Design review of the part built by this model. Coordinates are the model's own, in mm. Coordinates: 2 decimals unless noted, no trailing zeros. Loops run counter-clockwise (first coordinate to the right, second up) from the corner with the lowest first, then second, coordinate; pieces in that order, holes last. Notation, with made-up numbers: M 84,65 L 143,65 A19 cw 143,82 Z; hole C -4.5,-18 d7. An arc over 180 degrees is marked long. One line per item, written item: value.
```python
from build123d import *

# Parameters (mm, degrees)
EXTRUDE_1_DEPTH     = 2
SKETCH_3_W          = 2
SKETCH_3_H          = 5
CUT_EXTRUDE_2_DEPTH = 10
CHAMFER_1_SIZE      = 3
SKETCH_4_W          = 16
SKETCH_4_H          = 3
CUT_EXTRUDE_3_DEPTH = 2
FILLET_1_R          = 1
FILLET_START        = -1
FILLET_2_DEPTH      = 4
FILLET_2_2_DEPTH    = 2
FILLET_3_R          = 0.5
CUT_EXTRUDE_4_DEPTH = 10
SKETCH_7_R          = 1
CUT_EXTRUDE_6_DEPTH = 10
FILLET_5_R          = 1


with BuildPart() as part:
    # 草图1 → 凸台-拉伸1 (new body)
    with BuildSketch(Plane(origin=(0, 0, 0), x_dir=(1, 0, 0), z_dir=(0, 1, 0))):
        Polygon((40, -10), (40, 0), (0, 0), (0, 5), (47.2, 5), (47.2, 0), (47.2, -10), align=None)
    extrude_1 = extrude(amount=EXTRUDE_1_DEPTH)

    # 草图3 → 切除-拉伸2 (cut)
    with BuildSketch(Plane.XZ):
        with Locations((41, 7.5)):
            Rectangle(SKETCH_3_W, SKETCH_3_H)
    cut_extrude_2 = extrude(amount=-CUT_EXTRUDE_2_DEPTH, mode=Mode.SUBTRACT)

    # 镜向1: 凸台-拉伸1, 切除-拉伸2 across plane
    add(extrude_1.mirror(Plane(origin=(0, 0, 0), x_dir=(0, 0, 1), z_dir=(1, 0, 0))))
    add(cut_extrude_2.mirror(Plane(origin=(0, 0, 0), x_dir=(0, 0, 1), z_dir=(1, 0, 0))), mode=Mode.SUBTRACT)

    # 倒角1
    chamfer_1_edges = [part.edges().sort_by_distance(p)[0] for p in [
        (47.2, 1, -5),
        (-47.2, 1, -5),
    ]]
    chamfer(chamfer_1_edges, length=CHAMFER_1_SIZE)

    # 草图4 → 切除-拉伸3 (cut)
    with BuildSketch(Plane.XZ):
        Rectangle(SKETCH_4_W, SKETCH_4_H)
    extrude(amount=-CUT_EXTRUDE_3_DEPTH, mode=Mode.SUBTRACT)

    # 圆角1
    fillet_1_edges = [part.edges().sort_by_distance(p)[0] for p in [
        (-8, 1, -1.5),
        (8, 1, -1.5),
    ]]
    fillet(fillet_1_edges, radius=FILLET_1_R)

    # 圆角2: read off the stored shape, not the designer's step
    # 圆角2 outline → 圆角2 (cut)
    with BuildSketch(Plane(origin=(0, 0, 0), x_dir=(1, 0, 0), z_dir=(0, 1, 0)).offset(FILLET_START)):
        with BuildLine():
            Line((-40, -5), (-40, -4))
            ThreePointArc((-40, -4), (-40.292893219, -4.707106781), (-41, -5))
            Line((-41, -5), (-40, -5))
        make_face()
        with BuildLine():
            Line((40, -5), (41, -5))
            ThreePointArc((41, -5), (40.292893219, -4.707106781), (40, -4))
            Line((40, -4), (40, -5))
        make_face()
    extrude(amount=FILLET_2_DEPTH, mode=Mode.SUBTRACT)

    # Fillet 2 2 outline → Fillet 2 2 (add)
    with BuildSketch(Plane(origin=(0, 0, 0), x_dir=(1, 0, 0), z_dir=(0, 1, 0))):
        with BuildLine():
            ThreePointArc((-42, -6), (-41.707106781, -5.292893219), (-41, -5))
            Line((-41, -5), (-42, -5))
            Line((-42, -5), (-42, -6))
        make_face()
        with BuildLine():
            ThreePointArc((41, -5), (41.707106781, -5.292893219), (42, -6))
            Line((42, -6), (42, -5))
            Line((42, -5), (41, -5))
        make_face()
    extrude(amount=FILLET_2_2_DEPTH)

    # 圆角3
    fillet_3_edges = [part.edges().sort_by_distance(p)[0] for p in [
        (47.2, 1, 10),
        (42, 1, 10),
        (-47.2, 1, 10),
        (-42, 1, 10),
    ]]
    fillet(fillet_3_edges, radius=FILLET_3_R)

    # 草图5 → 切除-拉伸4 (cut)
    with BuildSketch(Plane.XZ):
        with BuildLine():
            Line((43.6, 1.5), (43.6, 7.5))
            ThreePointArc((43.6, 7.5), (44.6, 8.5), (45.6, 7.5))
            Line((45.6, 7.5), (45.6, 1.5))
            ThreePointArc((45.6, 1.5), (44.6, 0.5), (43.6, 1.5))
        make_face()
    cut_extrude_4 = extrude(amount=-CUT_EXTRUDE_4_DEPTH, mode=Mode.SUBTRACT)

    # 镜向2: 切除-拉伸4 across plane
    add(cut_extrude_4.mirror(Plane(origin=(0, 0, 0), x_dir=(0, 0, 1), z_dir=(1, 0, 0))), mode=Mode.SUBTRACT)

    # 草图7 → 切除-拉伸6 (cut)
    with BuildSketch(Plane.XZ):
        with Locations((40, 1)):
            Circle(SKETCH_7_R)
        with Locations((-40, 1)):
            Circle(SKETCH_7_R)
    extrude(amount=-CUT_EXTRUDE_6_DEPTH, mode=Mode.SUBTRACT)

    # 圆角5
    fillet_5_edges = [part.edges().sort_by_distance(p)[0] for p in [
        (40, 1, 2),
        (-40, 1, 2),
    ]]
    fillet(fillet_5_edges, radius=FILLET_5_R)


solid = part.part
```
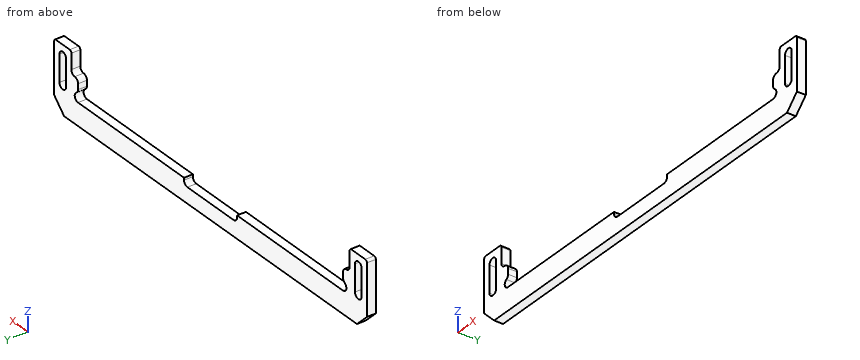
(1) To check wall thickness, follow line 1 along X through (y, z) = (1.8, 6.75); line 2 along X through (y, z) = (1.95, 1.5); line 3 along Z through (x, y) = (32, 1.3). State the ranges of each line that lie inside material, in increasing order. Write a range as [from, to].
Reply:
line 1: x = [-47.2, -45.6], [-43.6, -42], [42, 43.6], [45.6, 47.2]
line 2: x = [-47.2, -45.6], [-43.6, -40.87], [40.87, 43.6], [45.6, 47.2]
line 3: z = [-5, 0]
(2) We need section A-A on z = -3.25. State the section outline as (x, y) points, then the cut area to 3 significant figures.
Reply:
outline: M -45.95,0 L 45.95,0 L 45.95,2 L -45.95,2 Z
area: 184 mm2
(3) Insertion check: pin 1 (0.6 mm diameter, centred on x = 2.5, y = 1.5, fed in from +Z). The pin has a flat end and moves straight along its axis. Give the tip position at first contact, or say it passes through.
Reply:
pin 1: stops at z = -1.5
(4) We need section C-C on x = 1.5. State the section outline as (y, z) points.
Reply:
outline: M 0,-5 L 2,-5 L 2,-1.5 L 0,-1.5 Z
(5) We need section B-B on y = 0.4. State how many separate pieces and enclosed holes the cut face has, then the cut area to 3 significant figures.
Reply:
separate pieces: 1
enclosed holes: 2
area: 530 mm2
